Here's how the part is built. I have some questions about the finished solid (model axes, mm). A direction names the side the tool comes from. Round coordinates to 2 decimals unless told otherwise and drop trailing zeros. Order: outer loops, then holes, each group sorted by start corner. A loop starts at its lowest first (then second) coordinate and runs counter-clockwise, first axis right, second up.
```python
from build123d import *

# Parameters (mm, degrees)
SKETCH_W        = 147
SKETCH_H        = 20
PAD_DEPTH       = 13
SKETCH001_W     = 16
SKETCH001_H     = 20
POCKET_DEPTH    = 10
SKETCH002_W     = 20
SKETCH002_H     = 13
PAD001_DEPTH    = 60
SKETCH003_R     = 3.5
POCKET001_DEPTH = 13.001


with BuildPart() as part:
    # Sketch → Pad (new body)
    with BuildSketch(Plane.XY):
        with Locations((73.5, 10)):
            Rectangle(SKETCH_W, SKETCH_H)
    extrude(amount=PAD_DEPTH)

    # Sketch001 (on Face6 of Pad) → Pocket (cut)
    with BuildSketch(Plane.XY.offset(13)):
        with Locations((13, 10)):
            Rectangle(SKETCH001_W, SKETCH001_H)
        with Locations((134, 10)):
            Rectangle(SKETCH001_W, SKETCH001_H)
    extrude(amount=-POCKET_DEPTH, mode=Mode.SUBTRACT)

    # Sketch002 (on Face14 of Pocket) → Pad001 (join)
    with BuildSketch(Plane(origin=(0, 20, 0), x_dir=(-1, 0, 0), z_dir=(0, 1, 0))):
        with Locations((-73.5, 6.5)):
            Rectangle(SKETCH002_W, SKETCH002_H)
    extrude(amount=PAD001_DEPTH)

    # Sketch003 (on Face17 of Pad001) → Pocket001 (cut, through all)
    with BuildSketch(Plane.XY.offset(13)):
        with Locations((73.5, 70)):
            Circle(SKETCH003_R)
    extrude(amount=-POCKET001_DEPTH, mode=Mode.SUBTRACT)


solid = part.part
```
1. If we mould it in two halves opening along X, with no side actions, what happens to faces 1 (the flat face through (38, 20, 6)), 2 (the flat face through (142, 10, 8)), 3 (the flat face through (63.5, 50, 6))? For each: released by +X, released by -X, zero draft, split by the parting line, or undercut.
Evaluation:
face 1: zero draft
face 2: undercut
face 3: released by -X
2. If we section it at C-C, the plane y = 70: Write out the boundary of the cut face in (x, z), and give its area (3 significant figures).
Evaluation:
outline: (63.5, 0) - (70, 0) - (70, 13) - (63.5, 13) - close; (77, 0) - (83.5, 0) - (83.5, 13) - (77, 13) - close
area: 169 mm2
3. I need wall thicknesses on probe 1 along X at (y, z) = (6.5, 9); probe 2 along Y at (x, z) = (73.5, 3.25); probe 3 along X at (y, z) = (30.5, 8.5). Which ranges of each line are inside material? Lowest first, please.
Evaluation:
probe 1: x = 0 to 5, 21 to 126, 142 to 147
probe 2: y = 0 to 66.5, 73.5 to 80
probe 3: x = 63.5 to 83.5
4. If we section it at A-A, the plane z = 5.5: Write out the boundary of the cut face in (x, y).
Evaluation:
outline: (0, 0) - (5, 0) - (5, 20) - (0, 20) - close; (21, 0) - (126, 0) - (126, 20) - (83.5, 20) - (83.5, 80) - (63.5, 80) - (63.5, 20) - (21, 20) - close; (142, 0) - (147, 0) - (147, 20) - (142, 20) - close; hole circle Ø7 at (73.5, 70)
5. If we section it at D-D, the plane x = 92: Write out the boundary of the cut face in (y, z), and give its area (3 significant figures).
Evaluation:
outline: (0, 0) - (20, 0) - (20, 13) - (0, 13) - close
area: 260 mm2
6. On a 3-axis mill with a long thin cutter (end or side, diameter ignored), from which of +Z, -Z, +X, -X, +Y, -Y can I reach the whole of each face in a straight line? I mean faces 4 (the flat face through (72, 0, 6)), 5 (the flat face through (83.5, 50, 6)), 6 (the flat face through (5, 10, 8)). Say none if no direction works.
Evaluation:
face 4: +Z, -Z, +X, -X, -Y
face 5: +Z, -Z, +X, +Y
face 6: +Z, +Y, -Y
7. I'm going to push flat-ended pins straight in: P1, Ø2, axis at x = 90.5, z = 11, coming from the +Y side; P2, Ø17.5, axis at x = 137, y = 11.5, coming from the +Z side; P3, Ø5, axis at y = 26, z = 5.5, coming from the -X side; P4, Ø1.5, axis at x = 19.5, z = 7.5, coming from the -Y side. Where does each tip first touch, or does it pass through?
Evaluation:
P1: stops at y = 20
P2: stops at z = 13
P3: stops at x = 63.5
P4: passes through
8. If we section it at B-B, the plane x = 73.5: Write out the boundary of the cut face in (y, z).
Evaluation:
outline: (0, 0) - (66.5, 0) - (66.5, 13) - (0, 13) - close; (73.5, 0) - (80, 0) - (80, 13) - (73.5, 13) - close
